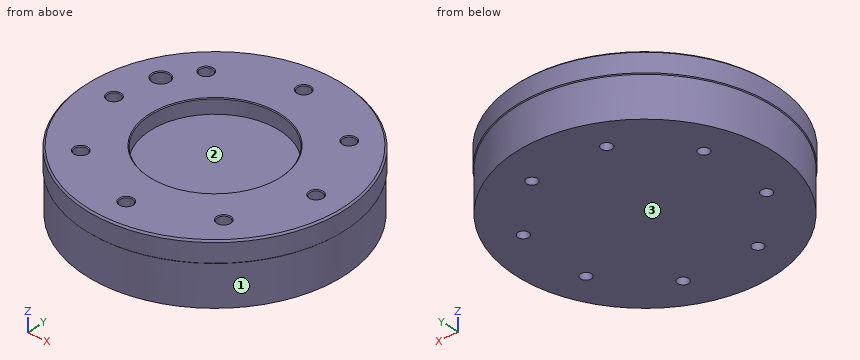
Autodesk Inventor part; units mm, degrees
ref_plane "YZ Plane" through (0, 0, 0) normal (1, 0, 0) x (0, 1, 0)
ref_plane "XZ Plane" through (0, 0, 0) normal (0, 1, 0) x (-1, 0, 0)
ref_plane "XY Plane" through (0, 0, 0) normal (0, 0, 1) x (1, 0, 0)
sketch "Sketch2" plane through (0, 0, 0) normal (1, 0, 0) x (0, 1, 0)
  line L0 (-80, 38) -> (0, 38)
  line L1 (-80, 38) -> (-80, 25.5)
  line L2 (-80, 25.5) -> (-79.5, 25)
  line L3 (-79.5, 25) -> (-79.5, 0)
  line L4 (-79.5, 0) -> (0, 0)
  line L5 (0, 38) -> (0, 0)
  line L6 (0, 0) -> (0, 10)
revolve "Revolve1" add sketch "Sketch2" angle 360 about axis through (0, 0, 0) along (0, 0, 1)
sketch "Sketch4" plane through (0, 0, 38) normal (0, 0, 1) x (1, 0, 0)
  circle A0 centre (0, 0) radius 80
  circle A1 centre (0, 0) radius 62.5 construction
  circle A2 centre (0, 0) radius 80
  point P0 (0, 62.5)
  dimension "d12" = 125
hole "Hole2" at (0, 62.5, 38) direction (0, 0, -1) diameter 7.798 depth 25 tip angle 118
pattern_circular "Circular Pattern1" count 8 over 360 about axis through (0, 0, 31.75) along (0, 0, 1) of "Hole2"
chamfer "Chamfer1" distance 1 angle 45 1 edges at (0, 80, 38)
sketch "Sketch3" plane through (0, 0, 38) normal (0, 0, 1) x (1, 0, 0)
  point P0 (0, 0)
hole "Hole1" at (0, 0, 38) direction (0, 0, -1) diameter 80 depth 9
chamfer "Chamfer2" distance 0.5 angle 45 9 edges at (-46.9512, 46.9512, 38) (-66.399, 0, 38) (-46.9512, -46.9512, 38) (0, -66.399, 38) (46.9512, -46.9512, 38) (66.399, 0, 38) (46.9512, 46.9512, 38) (0, 66.399, 38) (0, 40, 38)
sketch "Sketch5" plane through (0, 0, 38) normal (0, 0, 1) x (1, 0, 0)
  circle A0 centre (-44.1942, 44.1942) radius 4.399
  circle A1 centre (0, 0) radius 40.5
  circle A2 centre (0, 62.5) radius 4.399
  circle A3 centre (-62.5, 0) radius 4.399
  arc A4 (-44.1942, 44.1942) -> (-62.5, 0) centre (0, 0) ccw construction
  line L0 (0, 0) -> (0, 62.5) construction
  line L1 (0, 0) -> (-56.6442, 26.4136) construction
  dimension "d25" = 65
hole "Hole3" at (-56.6442, 26.4136, 38) direction (0, 0, -1) diameter 10.106 depth 15 tip angle 118
chamfer "Chamfer3" distance 0.5 angle 45 1 edges at (-56.6442, 31.4666, 38)
sketch "Sketch6" plane through (0, 0, 0) normal (0, 0, -1) x (-1, 0, 0)
  circle A0 centre (0, 0) radius 79.5
  circle A1 centre (0, 0) radius 59.2292
  point P0 (-54.1926, 23.901)
hole "Hole4" at (54.1926, 23.901, 0) direction (0, 0, 1) diameter 6.647 depth 12 tip angle 118
pattern_circular "Circular Pattern2" count 8 over 360 about axis through (0, 0, 12.5) along (0, 0, 1) of "Hole4"
properties part number "100022" material "STEEL - HIGH GRADE ALLOY, BLACK OXIDE FINISH"
Could you check a few things on this model? Use its own coordinates, in mm. Face numbers are marked on the shaded views. Coordinates: 2 decimals unless noted, no trailing zeros. Use one line per item in the form item = value. Start each with the question number.
1. For pin 1 (4 mm diameter, centred on x = 54.19, y = 23.9, fed in from -Z); pin 2 (8.5 mm diameter, centred on x = 23.9, y = -54.19, fed in from -Z); pin 3 (4 mm diameter, centred on y = 59, z = 26, fed in from -X); pin 4 (6 mm diameter, centred on x = 0, y = 62.5, fed in from +Z), each with a flat end and sliding along its axis, tell me the tip position at first contact or that it passes through.
2. We'd pull the mould along Y, two halves only. Please class the marked faces 1, 2 and 3: +Y half, -Y half, draft (parallel to the pull), parting line (faces both ways), or undercut.
3. Suppose I cut it at A-A on z = 16. Count the separate pieces of the cut face and the enclosed holes in it, then the cut area to 3 significant figures.
4. Please list where these lines run through material, in increasing order: line 1 (Y direction, x = 45.5, z = 20.5); line 2 (X direction, y = -3.5, z = 18); line 3 (Z direction, x = 15, y = -15.5).
Geometry says:
q1.pin_1 = 12.79
q1.pin_2 = 0
q1.pin_3 = -56.13
q1.pin_4 = 12.46
q2.face_1 = parting line
q2.face_2 = undercut
q2.face_3 = draft
q3.separate_pieces = 1
q3.enclosed_holes = 8
q3.area = 19,500 mm^2
q4.line_1 = -65.19 to -47.87, -40.52 to 40.52, 47.87 to 65.19
q4.line_2 = -79.42 to -64.22, -60.78 to 60.78, 64.22 to 79.42
q4.line_3 = 0 to 29
